```python
from build123d import *

# Parameters (mm, degrees)
SKETCH3_W                = 6.35
SKETCH3_H                = 6.88975
BOSS_EXTRUDE3_DEPTH      = 2.921
FILLET1_R                = 2.54
BOSS_EXTRUDE5_DEPTH      = 3.429
BOSS_EXTRUDE5_DEPTH_BACK = 9.779
SKETCH5_W                = 1.190625
SKETCH5_H                = 1.1350625
FILLET7_START            = 1.4605
FILLET7_DEPTH            = 1.984375
FILLET7_START_2          = -4.6355
FILLET7_2_DEPTH          = 6.096
FILLET7_START_3          = -3.175
FILLET7_3_DEPTH          = 0.733117551
FILLET7_START_4          = 2.441882449
FILLET7_4_DEPTH          = 0.733117551
FILLET7_START_5          = -3.4448751
FILLET7_5_DEPTH          = 4.9053751
FILLET8_R                = 1.27
FILLET10_R               = 0.635
SKETCH6_W                = 2.54
SKETCH6_H                = 1.905
CUT_EXTRUDE1_DEPTH       = 2.032


with BuildPart() as part:
    # Sketch3 → Boss-Extrude3 (new body)
    with BuildSketch(Plane(origin=(0, 0, 0), x_dir=(1, 0, 0), z_dir=(0, 1, 0))):
        Rectangle(SKETCH3_W, SKETCH3_H)
    extrude(amount=BOSS_EXTRUDE3_DEPTH)

    # Fillet1
    fillet1_edges = [part.edges().sort_by_distance(p)[0] for p in [
        (0, 2.921, 3.444875),
    ]]
    fillet(fillet1_edges, radius=FILLET1_R)

    # Sketch5 → Boss-Extrude5 (add, two sides: drawn at the far end of the back side and taken through both)
    with BuildSketch(Plane.ZY.offset(3.175).offset(-BOSS_EXTRUDE5_DEPTH_BACK)):
        with BuildLine():
            Line((-3.444875, 0), (1.4605, 0))
            Line((1.4605, 0), (1.4605, 0.1190625))
            ThreePointArc((1.4605, 0.1190625), (1.16292049, 0.83748299), (0.4445, 1.1350625))
            Line((0.4445, 1.1350625), (-3.444875, 1.1350625))
            Line((-3.444875, 1.1350625), (-3.444875, 0))
        make_face()
        with Locations((-4.0401875, 0.56753125)):
            Rectangle(SKETCH5_W, SKETCH5_H)
    extrude(amount=BOSS_EXTRUDE5_DEPTH + BOSS_EXTRUDE5_DEPTH_BACK)

    # Fillet7: read off the stored shape, not the designer's step
    # Fillet7 outline → Fillet7 (cut)
    with BuildSketch(Plane.XY.offset(FILLET7_START)):
        with BuildLine():
            Line((1.905, 0), (3.175, 0))
            Line((3.175, 0), (3.175, 1.27))
            ThreePointArc((3.175, 1.27), (2.803025612, 0.371974388), (1.905, 0))
        make_face()
        with BuildLine():
            Line((-3.175, 0), (-1.905, 0))
            ThreePointArc((-1.905, 0), (-2.803025612, 0.371974388), (-3.175, 1.27))
            Line((-3.175, 1.27), (-3.175, 0))
        make_face()
    extrude(amount=FILLET7_DEPTH, mode=Mode.SUBTRACT)

    # Fillet7 2 outline → Fillet7 2 (cut)
    with BuildSketch(Plane.XY.offset(FILLET7_START_2)):
        with BuildLine():
            ThreePointArc((3.175, 1.27), (3.173201501, 1.202435569), (3.167811099, 1.1350625))
            Line((3.167811099, 1.1350625), (3.175, 1.1350625))
            Line((3.175, 1.1350625), (3.175, 1.27))
        make_face()
        with BuildLine():
            Line((-3.175, 1.1350625), (-3.167811099, 1.1350625))
            ThreePointArc((-3.167811099, 1.1350625), (-3.173201501, 1.202435569), (-3.175, 1.27))
            Line((-3.175, 1.27), (-3.175, 1.1350625))
        make_face()
    extrude(amount=FILLET7_2_DEPTH, mode=Mode.SUBTRACT)

    # Fillet7 3 outline → Fillet7 3 (cut)
    with BuildSketch(Plane.YZ.offset(FILLET7_START_3)):
        with BuildLine():
            Line((1.1350625, 1.4605), (0.1190625, 1.4605))
            ThreePointArc((0.1190625, 1.4605), (0.83748299, 1.16292049), (1.1350625, 0.4445))
            Line((1.1350625, 0.4445), (1.1350625, 1.4605))
        make_face()
    extrude(amount=FILLET7_3_DEPTH, mode=Mode.SUBTRACT)

    # Fillet7 4 outline → Fillet7 4 (cut)
    with BuildSketch(Plane.YZ.offset(FILLET7_START_4)):
        with BuildLine():
            Line((1.1350625, 1.4605), (0.1190625, 1.4605))
            ThreePointArc((0.1190625, 1.4605), (0.83748299, 1.16292049), (1.1350625, 0.4445))
            Line((1.1350625, 0.4445), (1.1350625, 1.4605))
        make_face()
    extrude(amount=FILLET7_4_DEPTH, mode=Mode.SUBTRACT)

    # Fillet7 5 outline → Fillet7 5 (add)
    with BuildSketch(Plane.XY.offset(FILLET7_START_5)):
        with BuildLine():
            Line((2.441882449, 1.1350625), (2.441882467, 0.119062462))
            ThreePointArc((2.441882467, 0.119062462), (2.938338401, 0.531683166), (3.167811099, 1.1350625))
            Line((3.167811099, 1.1350625), (2.441882449, 1.1350625))
        make_face()
        with BuildLine():
            ThreePointArc((-3.167811099, 1.1350625), (-2.938338401, 0.531683166), (-2.441882467, 0.119062462))
            Line((-2.441882467, 0.119062462), (-2.441882449, 1.1350625))
            Line((-2.441882449, 1.1350625), (-3.167811099, 1.1350625))
        make_face()
    extrude(amount=FILLET7_5_DEPTH)

    # Fillet8
    # the kernel refuses this fillet: 1.27 mm, written as the material it takes off along each edge
    with BuildSketch(Plane(origin=(-3.175, -1.905, -3.444875), x_dir=(0, 0, 1), z_dir=(0, 1, 0))) as fillet8_piece_1_section:
        with BuildLine():
            CenterArc((FILLET8_R, FILLET8_R), FILLET8_R, 180, 90)
            Line((0, FILLET8_R), (0, 0))
            Line((0, 0), (FILLET8_R, 0))
        make_face()
    fillet8_piece_1 = extrude(amount=8.001, mode=Mode.PRIVATE)
    fillet8_piece_1 = split(fillet8_piece_1, bisect_by=Plane(origin=(-3.175, 1.1350625, -3.444875), z_dir=(0, 1, 0)), keep=Keep.TOP, mode=Mode.PRIVATE)
    add(fillet8_piece_1, mode=Mode.SUBTRACT)
    with BuildSketch(Plane(origin=(3.175, -1.905, -3.444875), x_dir=(-1, 0, 0), z_dir=(0, 1, 0))) as fillet8_piece_2_section:
        with BuildLine():
            CenterArc((FILLET8_R, FILLET8_R), FILLET8_R, 180, 90)
            Line((0, FILLET8_R), (0, 0))
            Line((0, 0), (FILLET8_R, 0))
        make_face()
    fillet8_piece_2 = extrude(amount=8.001, mode=Mode.PRIVATE)
    fillet8_piece_2 = split(fillet8_piece_2, bisect_by=Plane(origin=(3.175, 1.1350625, -3.444875), z_dir=(0, 1, 0)), keep=Keep.TOP, mode=Mode.PRIVATE)
    add(fillet8_piece_2, mode=Mode.SUBTRACT)

    # Fillet10
    fillet10_edges = [part.edges().sort_by_distance(p)[0] for p in [
        (-6.604, 0.83748299, 1.16292049),
        (-6.604, 1.1350625, -2.0955),
        (-6.604, 0.05953125, 1.4605),
        (6.604, 0.83748299, 1.16292049),
        (6.604, 0.05953125, 1.4605),
        (6.604, 1.1350625, -2.0955),
    ]]
    fillet(fillet10_edges, radius=FILLET10_R)

    # Sketch6 → Cut-Extrude1 (cut)
    with BuildSketch(Plane.XZ):
        with Locations((0, -1.2065)):
            Rectangle(SKETCH6_W, SKETCH6_H)
    extrude(amount=-CUT_EXTRUDE1_DEPTH, mode=Mode.SUBTRACT)


solid = part.part
```
Here's how the part is built. I have some questions about the finished solid (model axes, mm). A direction names the side the tool comes from. Give positions to 0.01 mm unless a question says otherwise; leave off trailing zeros. Order: outer loops, then holes, each group sorted by start corner. A loop starts at its lowest first (then second) coordinate and runs counter-clockwise, first axis right, second up. Notation, with made-up numbers: (71, 28) -> (92, 28) arc R11 cw to (92, 38) -> close; hole circle Ø7 at (55, 4.25). An arc over 180 degrees is marked (long way). Use CSV: the item, a comma, the result in double quotes. Start each with the question number.
Item 1: Suppose I cut it at A-A (z = 0.25). List the corners of the cut face in (x, y) for me (3 decimals).
Item 2: Thinking about a two-plate mould opening in Z: for faces 1 (the flat face through (0, 1, -0.254)), 2 (the flat face through (-3.175, 2, 1)), 3 (the cylindrical face through (-4.6, 0.8, 1.2)), 4 (the flat face through (1.27, 1, -1)), which applies, pulls with the +Z half, pulls with the -Z half, needs draft (parallel to the pull), parting line crosses it, or undercut?
Item 3: Suppose I cut it at B-B (x = 0.75). List the corners of the cut face in (y, z) for me, and give its area (3 significant figures).
Item 4: If I drill on probe 1 along X at (y, z) = (0.45, -1.75); probe 2 along X at (y, z) = (1.7, 1) (3 decimals); probe 3 along Z at (x, y) = (-3, 0.1), over which ranges is the centre line in solid material (lowest first)? Write a range as [from, to].
Item 5: Suppose I cut it at D-D (z = -1.5). List the corners of the cut face in (x, y) for me (3 decimals), and give its area (3 significant figures).
Item 6: On a 3-axis mill with a long thin cutter (end or side, diameter ignored), from which of +Z, -Z, +X, -X, +Y, -Y can I reach the whole of each face in a straight line? I mean faces 5 (the flat face through (0, 2, -3.445)), 6 (the flat face through (3.175, 2, 1)), 7 (the cylindrical face through (2.813, 2.016, -3.063)), 8 (the flat face through (0, 2.032, -1)). Say none if no direction works.
Item 7: I'm going to push flat-ended pins straight in: P1, Ø1, axis at x = -0.5, y = 1, coming from the +Z side; P2, Ø1, axis at x = 3.5, z = 2.5, coming from the +Y side; P3, Ø1.5, axis at y = 1, z = -1, coming from the +X side; P4, Ø1, axis at x = -0.5, z = -1, coming from the -Y side. Where does each tip first touch, or does it pass through?
Item 8: Suppose I cut it at C-C (y = 1.65). List the corners of the cut face in (x, z) for me (3 decimals).
Answer block:
1,outline,"(-6.604, 0) -> (6.604, 0) -> (6.604, 0.5) arc R0.635 ccw to (5.969, 1.135) -> (3.168, 1.135) arc R1.27 ccw to (3.175, 1.27) -> (3.175, 2.921) -> (-3.175, 2.921) -> (-3.175, 1.27) arc R1.27 ccw to (-3.168, 1.135) -> (-5.969, 1.135) arc R0.635 ccw to (-6.604, 0.5) -> close"
2,face 1,"undercut"
2,face 2,"needs draft"
2,face 3,"pulls with the +Z half"
2,face 4,"undercut"
3,outline,"(0, -4.64) -> (1.14, -4.64) -> (1.14, -3.44) -> (2.92, -3.44) -> (2.92, 0.9) arc R2.54 ccw to (0.38, 3.44) -> (0, 3.44) -> (0, -0.25) -> (2.03, -0.25) -> (2.03, -2.16) -> (0, -2.16) -> close"
3,area,"16.2 mm^2"
4,probe 1,"x = [-6.6, -1.27], [1.27, 6.6]"
4,probe 2,"x = [-3.175, 3.175]"
4,probe 3,"z = [-4.64, 1.46]"
5,outline,"(-6.604, 0) -> (-1.27, 0) -> (-1.27, 2.032) -> (1.27, 2.032) -> (1.27, 0) -> (6.604, 0) -> (6.604, 0.5) arc R0.635 ccw to (5.969, 1.135) -> (3.168, 1.135) arc R1.27 ccw to (3.175, 1.27) -> (3.175, 2.921) -> (-3.175, 2.921) -> (-3.175, 1.27) arc R1.27 ccw to (-3.168, 1.135) -> (-5.969, 1.135) arc R0.635 ccw to (-6.604, 0.5) -> close"
5,area,"21.0 mm^2"
6,face 5,"-Z, +X, -X, +Y"
6,face 6,"+Z, -Z, +X, +Y"
6,face 7,"-Z, +X, +Y"
6,face 8,"-Y"
7,P1,"stops at z = 3.44"
7,P2,"stops at y = 2.61"
7,P3,"stops at x = 6.6"
7,P4,"stops at y = 2.03"
8,outline,"(-3.175, -2.175) arc R1.27 ccw to (-1.905, -3.445) -> (1.905, -3.445) arc R1.27 ccw to (3.175, -2.175) -> (3.175, 3.105) -> (-3.175, 3.105) -> close; hole (-1.27, -2.159) -> (1.27, -2.159) -> (1.27, -0.254) -> (-1.27, -0.254) -> close"
